Can you work these out from the drawing? Everything is in mm from the part's minimum corner. A direction names the side the tool comes from. Give positions to 0.01 mm unless a question says otherwise; leave off trailing zeros. Loops run counter-clockwise (first coordinate to the right, second up) from the corner with the lowest first, then second, coordinate; pieces in that order, holes last. Notation, with made-up numbers: (36.25, 55) - (42.25, 55) arc R11 cw to (42.25, 69) - close; hole circle Ø7 at (24, -22). An arc over 180 degrees is marked (long way). Answer in a Markdown table with one row per item.
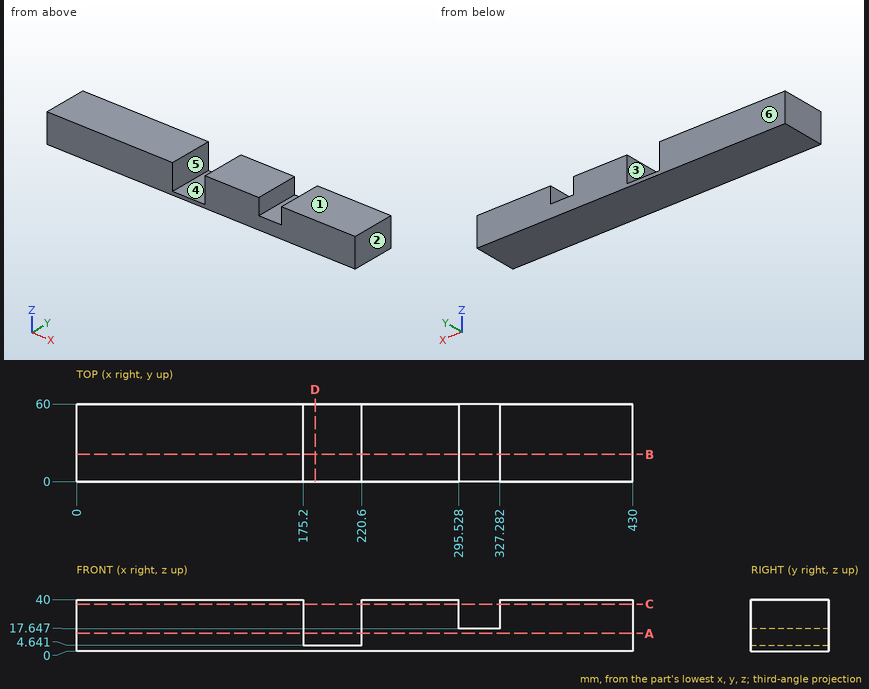
Q1. If we mould it in two halves opening along X, with no side actions, what happens to the marked faces 1, 2, 3 and 4? For each: released by +X, released by -X, zero draft, split by the parting line, or undercut.
Checked values:
| item | result |
|---|---|
| face 1 | zero draft |
| face 2 | released by +X |
| face 3 | undercut |
| face 4 | undercut |
Q2. On a 3-axis mill with a long thin cutter (end or side, diameter ignored), from which of +Z, -Z, +X, -X, +Y, -Y can I reach the whole of each face in a straight line? I mean the marked faces 5 and 6. Say none if no direction works.
Checked values:
| item | result |
|---|---|
| face 5 | +Z, +Y, -Y |
| face 6 | +Z, -Z, +X, -X, +Y |
Q3. Imagine slicing it at C-C, the plane z = 36.5. Write out the boundary of the cut face in (x, y), and give its area (3 significant figures).
Checked values:
| item | result |
|---|---|
| outline | (0, 0) - (175.2, 0) - (175.2, 60) - (0, 60) - close; (220.6, 0) - (295.53, 0) - (295.53, 60) - (220.6, 60) - close; (327.28, 0) - (430, 0) - (430, 60) - (327.28, 60) - close |
| area | 21,200 mm² |
Q4. Imagine slicing it at D-D, the plane x = 184.5. Write out the boundary of the cut face in (y, z).
Checked values:
| item | result |
|---|---|
| outline | (0, 0) - (60, 0) - (60, 4.64) - (0, 4.64) - close |
Q5. Imagine slicing it at B-B, the plane y = 21. Write out the boundary of the cut face in (x, z).
Checked values:
| item | result |
|---|---|
| outline | (0, 0) - (430, 0) - (430, 40) - (327.28, 40) - (327.28, 17.65) - (295.53, 17.65) - (295.53, 40) - (220.6, 40) - (220.6, 4.64) - (175.2, 4.64) - (175.2, 40) - (0, 40) - close |
Q6. If I drill on line 1 (X direction, y = 12, z = 33.5); line 2 (X direction, y = 24.5, z = 11.5); line 3 (Z direction, x = 315.5, y = 56.5), over which ranges is the centre line in solid material (lowest first)? Write a range as [from, to].
Checked values:
| item | result |
|---|---|
| line 1 | x = [0, 175.2], [220.6, 295.53], [327.28, 430] |
| line 2 | x = [0, 175.2], [220.6, 430] |
| line 3 | z = [0, 17.65] |
Q7. For pin 1 (1 mm diameter, centred on x = 220.5, z = 13.5, fed in from -Y); pin 2 (13.5 mm diameter, centred on x = 191, y = 21.5, fed in from +Z), each with a flat end and sliding along its axis, tell me the tip position at first contact or that it passes through.
Checked values:
| item | result |
|---|---|
| pin 1 | stops at y = 0 |
| pin 2 | stops at z = 4.64 |
Q8. Imagine slicing it at A-A, the plane z = 14. Write out the boundary of the cut face in (x, y), and give its area (3 significant figures).
Checked values:
| item | result |
|---|---|
| outline | (0, 0) - (175.2, 0) - (175.2, 60) - (0, 60) - close; (220.6, 0) - (430, 0) - (430, 60) - (220.6, 60) - close |
| area | 23,100 mm² |
